Source: CAD feature listing. Evaluate the final solid. Frame: model axes, mm. A direction names the side the tool comes from. Give positions to 0.01 mm unless a question says otherwise; leave off trailing zeros. Order: outer loops, then holes, each group sorted by start corner. A loop starts at its lowest first (then second) coordinate and runs counter-clockwise, first axis right, second up. Notation, with made-up numbers: (-35.75, -19.5) -> (18.25, -19.5) arc R20 cw to (18.25, 3.5) -> close; hole circle Ø2 at (87, 18). An arc over 180 degrees is marked (long way). Use CSV: the item, a comma, the result in double quotes.
```python
from build123d import *

# Parameters (mm, degrees)
BOSS_EXTRU_1_DEPTH      = 15.35
ESQUISSE2_W             = 12.15
ESQUISSE2_H             = 42.66
ENL_V_MAT_EXTRU_1_DEPTH = 53.912475845
CONG_1_R                = 1
ESQUISSE3_R             = 1.5
ENL_V_MAT_EXTRU_2_DEPTH = 53.912475845
ESQUISSE4_R             = 1.5
ENL_V_MAT_EXTRU_3_DEPTH = 53.912475845


with BuildPart() as part:
    # Esquisse1 → Boss.-Extru.1 (new body)
    with BuildSketch(Plane(origin=(0, 0, 0), x_dir=(0, 0, -1), z_dir=(1, 0, 0))):
        Polygon((0, 0), (0, 44.26), (-24.6, 44.26), (-13.3, 0), align=None)
    extrude(amount=BOSS_EXTRU_1_DEPTH)

    # Esquisse2 → Enlèv. mat.-Extru.1 (cut, through all)
    with BuildSketch(Plane(origin=(0, 0, 0), x_dir=(-1, 0, 0), z_dir=(0, 0, -1))):
        with Locations((-7.675, 21.33)):
            Rectangle(ESQUISSE2_W, ESQUISSE2_H)
    extrude(amount=-ENL_V_MAT_EXTRU_1_DEPTH, mode=Mode.SUBTRACT)

    # Congé1
    cong_1_edges = [part.edges().sort_by_distance(p)[0] for p in [
        (15.35, 44.26, 12.3),
        (0.8, 0, 13.3),
        (0.8, 0, 0),
        (0, 44.26, 12.3),
        (14.55, 0, 13.3),
        (14.55, 0, 0),
    ]]
    fillet(cong_1_edges, radius=CONG_1_R)

    # Esquisse3 → Enlèv. mat.-Extru.2 (cut, through all)
    with BuildSketch(Plane.ZY):
        with Locations((5.85, 6.46)):
            Circle(ESQUISSE3_R)
    extrude(amount=-ENL_V_MAT_EXTRU_2_DEPTH, mode=Mode.SUBTRACT)

    # Esquisse4 → Enlèv. mat.-Extru.3 (cut, through all)
    with BuildSketch(Plane(origin=(0, 44.26, 0), x_dir=(1, 0, 0), z_dir=(0, 1, 0))):
        with Locations(Location((7.331518895, -19.6, 0), (0, 0, 270))):
            Circle(ESQUISSE4_R)
    extrude(amount=-ENL_V_MAT_EXTRU_3_DEPTH, mode=Mode.SUBTRACT)


solid = part.part
```
1. Section query B-B on y = 39.5. Return loops of the section in (x, z), plus the area to 3 significant figures.
Answer below:
outline,"(0, 0) -> (1.6, 0) -> (1.6, 23.38) -> (0, 23.38) -> close; (13.75, 0) -> (15.35, 0) -> (15.35, 23.38) -> (13.75, 23.38) -> close"
area,"74.8 mm²"
2. Access query for faces 5 (the flat face through (14, 26, 0)), 6 (the flat face through (8, 42.66, 12)). Directions: +Z, -Z, +X, -X, +Y, -Y. A direction counts if a zero-diameter tool reaches every point of the face in a straight line with its end or side. Return the directions, or none.
Answer below:
face 5,"-Z, +X, -X, +Y, -Y"
face 6,"+Z, -Z, -Y"
3. Section query A-A on z = 5.85. Return loops of the section in (x, y), plus the area to 3 significant figures.
Answer below:
outline,"(0, 0) -> (1.6, 0) -> (1.6, 4.96) -> (0, 4.96) -> close; (0, 7.96) -> (1.6, 7.96) -> (1.6, 42.66) -> (13.75, 42.66) -> (13.75, 7.96) -> (15.35, 7.96) -> (15.35, 43.26) arc R1 ccw to (14.35, 44.26) -> (1, 44.26) arc R1 ccw to (0, 43.26) -> close; (13.75, 0) -> (15.35, 0) -> (15.35, 4.96) -> (13.75, 4.96) -> close"
area,"151 mm²"
4. Mould query, pull axis X, two halves, no side actions, for faces 1 (the cylindrical face through (6.42, 43.47, 18.41)), 2 (the flat face through (0, 22, 10)), 3 (the cylindrical face through (15.049, 43.975, 12.472)), 4 (the cylindrical face through (0.811, 0.205, 13.129)). Classes: released by +X, released by -X, zero draft, split by the parting line, or undercut.
Answer below:
face 1,"undercut"
face 2,"released by -X"
face 3,"released by +X"
face 4,"zero draft"
5. Section query D-D on y = 6.46. Return loops of the section in (x, z), plus the area to 3 significant figures.
Answer below:
outline,"(0, 0) -> (1.6, 0) -> (1.6, 4.35) -> (0, 4.35) -> close; (0, 7.35) -> (1.6, 7.35) -> (1.6, 14.95) -> (0, 14.95) -> close; (13.75, 0) -> (15.35, 0) -> (15.35, 4.35) -> (13.75, 4.35) -> close; (13.75, 7.35) -> (15.35, 7.35) -> (15.35, 14.95) -> (13.75, 14.95) -> close"
area,"38.2 mm²"
6. Section query C-C on z = 3.25. Return loops of the section in (x, y), plus the area to 3 significant figures.
Answer below:
outline,"(0, 0) -> (1.6, 0) -> (1.6, 42.66) -> (13.75, 42.66) -> (13.75, 0) -> (15.35, 0) -> (15.35, 43.26) arc R1 ccw to (14.35, 44.26) -> (1, 44.26) arc R1 ccw to (0, 43.26) -> close"
area,"161 mm²"
7. Ray query, line 1 along X through (y, z) = (29.5, 18); line 2 along Y through (x, z) = (14.8, 5.85); line 3 along Y through (x, z) = (2.25, 10). Return the intervals inside material, ascending.
Answer below:
line 1,"x = 0 to 1.6, 13.75 to 15.35"
line 2,"y = 0 to 4.96, 7.96 to 44.15"
line 3,"y = 42.66 to 44.26"
8. Pin query (flat end, axial travel): P1, Ø6, axis at x = 3.5, y = 20, coming from the +Z side; P2, Ø6, axis at x = 9.5, z = 11, coming from the -Y side. Return the tip coordinate at first contact, or that it passes through.
Answer below:
P1,"stops at z = 19"
P2,"stops at y = 42.66"
